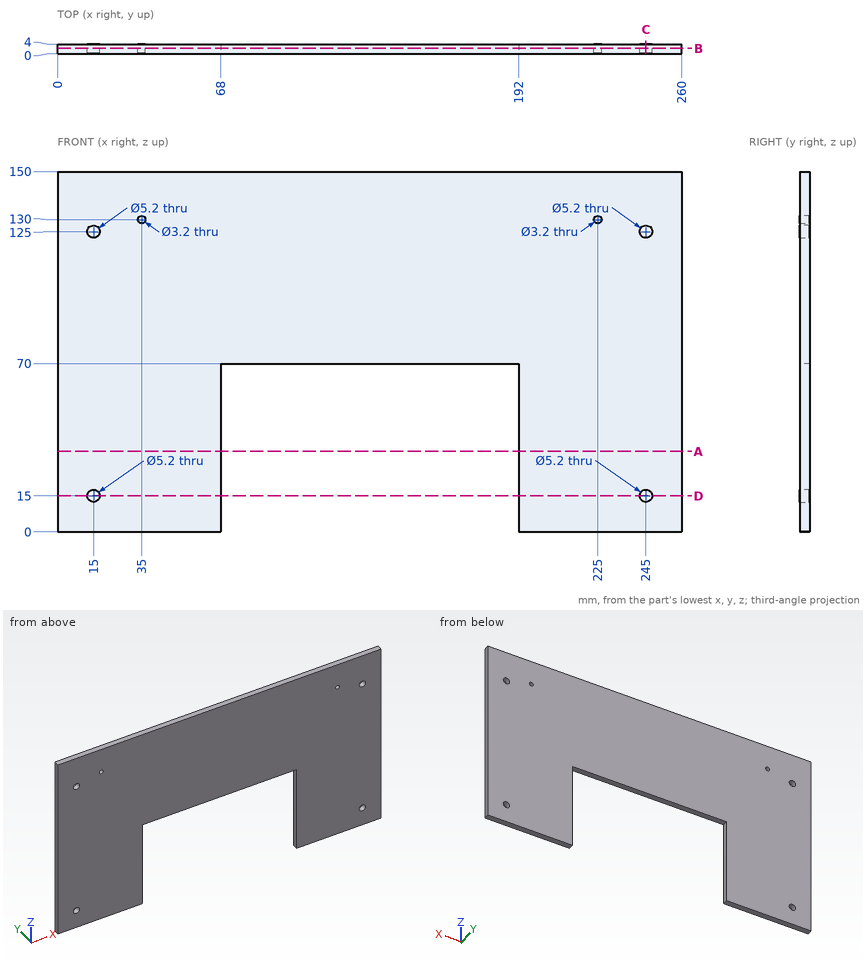
Geometry check sheet. Reference: drawing and pictorial views, mm from the part's lowest x, y, z. Coordinates: 2 decimals unless noted, no trailing zeros. Loops run counter-clockwise (first coordinate to the right, second up) from the corner with the lowest first, then second, coordinate; pieces in that order, holes last.
1) Material ranges on probe 1 along Z at (x, y) = (245, 3.1); probe 2 along X at (y, z) = (0.45, 10); probe 3 along X at (y, z) = (3.1, 125), recorded low to high.
2) Sectioned sample at B-B (y = 2.2). Record the boundary of the cut face in (x, z).
3) Gauge pin test, flat ends, axial feed: pin 1 (1.2 mm diameter, centred on x = 113, y = 2.5, fed in from -Z); pin 2 (2.5 mm diameter, centred on x = 35, z = 130, fed in from +Y). Record the tip position at first contact, or that the pin passes through.
4) Sectioned sample at C-C (x = 245). Record the boundary of the cut face in (y, z), and give its area (3 significant figures).
5) Sectioned sample at A-A (z = 33.5). Record the boundary of the cut face in (x, y), and give its area (3 significant figures).
6) Sectioned sample at D-D (z = 15). Record the boundary of the cut face in (x, y), and give its area (3 significant figures).
Check sheet entries:
1. probe 1: z = 0 to 12.4, 17.6 to 122.4, 127.6 to 150
1. probe 2: x = 0 to 68, 192 to 260
1. probe 3: x = 0 to 12.4, 17.6 to 242.4, 247.6 to 260
2. outline: (0, 0) - (68, 0) - (68, 70) - (192, 70) - (192, 0) - (260, 0) - (260, 150) - (0, 150) - close; hole circle Ø5.2 at (15, 15); hole circle Ø5.2 at (15, 125); hole circle Ø3.2 at (35, 130); hole circle Ø3.2 at (225, 130); hole circle Ø5.2 at (245, 15); hole circle Ø5.2 at (245, 125)
3. pin 1: stops at z = 70
3. pin 2: passes through
4. outline: (0, 0) - (4, 0) - (4, 12.4) - (0, 12.4) - close; (0, 17.6) - (4, 17.6) - (4, 122.4) - (0, 122.4) - close; (0, 127.6) - (4, 127.6) - (4, 150) - (0, 150) - close
4. area: 558 mm2
5. outline: (0, 0) - (68, 0) - (68, 4) - (0, 4) - close; (192, 0) - (260, 0) - (260, 4) - (192, 4) - close
5. area: 544 mm2
6. outline: (0, 0) - (12.4, 0) - (12.4, 4) - (0, 4) - close; (17.6, 0) - (68, 0) - (68, 4) - (17.6, 4) - close; (192, 0) - (242.4, 0) - (242.4, 4) - (192, 4) - close; (247.6, 0) - (260, 0) - (260, 4) - (247.6, 4) - close
6. area: 502 mm2
